```python
from build123d import *

# Parameters (mm, degrees)
BOSS_EXTRUDE1_DEPTH = 18
CUT_EXTRUDE1_DEPTH  = 14
SKETCH5_W           = 38.6
SKETCH5_H           = 4
BOSS_EXTRUDE2_DEPTH = 51.5
SKETCH6_R           = 10
CUT_EXTRUDE2_DEPTH  = 200
SKETCH7_R           = 6
CUT_EXTRUDE3_DEPTH  = 200


with BuildPart() as part:
    # Sketch2 → Boss-Extrude1 (new body)
    with BuildSketch(Plane(origin=(0, 0, 0), x_dir=(1, 0, 0), z_dir=(0, 1, 0))):
        with BuildLine():
            Line((-2.050203312, 17.379489819), (71.229085812, 26.024015225))
            Line((71.229085812, 26.024015225), (70.776256856, -26.027550211))
            Line((70.776256856, -26.027550211), (-2.063605293, -17.37790359))
            ThreePointArc((-2.063605293, -17.37790359), (-17.499998699, 0.006747763), (-2.050203312, 17.379489819))
        make_face()
    extrude(amount=BOSS_EXTRUDE1_DEPTH)

    # Sketch4 → Cut-Extrude1 (cut)
    with BuildSketch(Plane(origin=(0, 18, 0), x_dir=(1, 0, 0), z_dir=(0, 1, 0))):
        with BuildLine():
            Line((35.006766585, 14.999998474), (31.502988077, 14.586668832))
            ThreePointArc((31.502988077, 14.586668832), (20.004544926, -0.369225031), (32.22510993, -14.741098504))
            Line((32.22510993, -14.741098504), (34.245425362, -14.981008548))
            Line((34.245425362, -14.981008548), (70.834558469, -19.325924398))
            Line((70.834558469, -19.325924398), (71.170294461, 19.266095201))
            Line((71.170294461, 19.266095201), (35.006766585, 14.999998474))
        make_face()
    extrude(amount=-CUT_EXTRUDE1_DEPTH, mode=Mode.SUBTRACT)

    # Sketch5 → Boss-Extrude2 (add)
    with BuildSketch(Plane(origin=(70.997313391, 0, 0.617649806), x_dir=(0.008699293, 0, -0.99996216), z_dir=(0.99996216, 0, 0.008699293))):
        with Locations((0.591017469, 16)):
            Rectangle(SKETCH5_W, SKETCH5_H)
    extrude(amount=-BOSS_EXTRUDE2_DEPTH)

    # Sketch6 → Cut-Extrude2 (cut)
    with BuildSketch(Plane(origin=(0, 18, 0), x_dir=(1, 0, 0), z_dir=(0, 1, 0))):
        with Locations((2.500001301, 0)):
            Circle(SKETCH6_R)
    extrude(amount=-CUT_EXTRUDE2_DEPTH, mode=Mode.SUBTRACT)

    # Sketch7 → Cut-Extrude3 (cut)
    with BuildSketch(Plane(origin=(0, 18, 0), x_dir=(1, 0, 0), z_dir=(0, 1, 0))):
        with Locations((35.001789275, 0.053432271)):
            Circle(SKETCH7_R)
        with Locations((55.001789275, 0.053432271)):
            Circle(SKETCH7_R)
    extrude(amount=-CUT_EXTRUDE3_DEPTH, mode=Mode.SUBTRACT)


solid = part.part
```
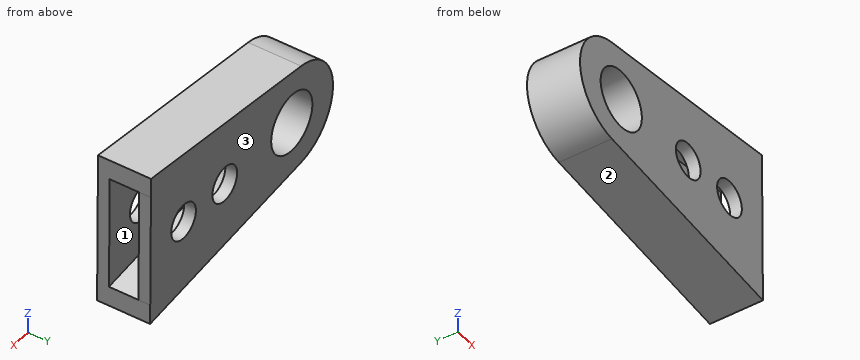
Read the model definition and answer for the solid it produces. Units are mm, in the model's axes. Face numbers are marked on the shaded views. Coordinates: 2 decimals unless noted, no trailing zeros. Loops run counter-clockwise (first coordinate to the right, second up) from the corner with the lowest first, then second, coordinate; pieces in that order, holes last. Notation, with made-up numbers: (60, 80.5) - (116, 80.5) arc R26 ccw to (116, 108.5) - close; hole circle Ø2 at (11, 88). An arc over 180 degrees is marked (long way). Answer in a Markdown table with one row per item.
1. Given pin 1 (8 mm diameter, centred on y = 4, z = 14, fed in from +X); pin 2 (10 mm diameter, centred on x = 36.5, y = 11.5, fed in from +Z); pin 3 (3 mm diameter, centred on x = 35.5, y = 3.5, fed in from +Z), each flat-ended and moving along its own axis, determine where each tip first touches the part or whether it passes through.
Conclusion:
| item | result |
|---|---|
| pin 1 | stops at x = 70.92 |
| pin 2 | stops at z = 22.55 |
| pin 3 | stops at z = 22.02 |
2. Find section C-C, the plane z = -1. Write down the section's boundary in (x, y), then the cut area to 3 significant figures.
Conclusion:
| item | result |
|---|---|
| outline | (-17.47, 0) - (-7.45, 0) - (-7.45, 18) - (-17.47, 18) - close; (12.45, 0) - (29.08, 0) - (29.08, 4) - (20.03, 4) - (20.03, 14) - (29.08, 14) - (29.08, 18) - (12.45, 18) - close; (40.93, 0) - (49.08, 0) - (49.08, 4) - (40.93, 4) - close; (40.93, 14) - (49.08, 14) - (49.08, 18) - (40.93, 18) - close; (60.93, 0) - (71.01, 0) - (71.01, 4) - (60.93, 4) - close; (60.93, 14) - (71.01, 14) - (71.01, 18) - (60.93, 18) - close |
| area | 535 mm² |
3. Find section D-D, the plane y = 15. Write down the section's boundary in (x, z), then the cut area to 3 significant figures.
Conclusion:
| item | result |
|---|---|
| outline | (-2.06, 17.38) arc R17.5 ccw to (-2.05, -17.38) - (71.23, -26.02) - (70.78, 26.03) - close; hole circle Ø20 at (2.5, 0); hole circle Ø12 at (35, -0.05); hole circle Ø12 at (55, -0.05) |
| area | 3,040 mm² |
4. Determine the mould class of the marked faces 1, 2 and 3 for opening direction Y: +Y half, -Y half, draft (parallel to the pull), parting line (faces both ways), or undercut.
Conclusion:
| item | result |
|---|---|
| face 1 | undercut |
| face 2 | draft |
| face 3 | +Y half |
5. Find section A-A, the plane y = 10.25. Write down the section's boundary in (x, z).
Conclusion:
| item | result |
|---|---|
| outline | (-2.06, 17.38) arc R17.5 ccw to (-2.05, -17.38) - (71.23, -26.02) - (71.17, -19.27) - (31.5, -14.59) arc R15 cw to (32.23, 14.74) - (70.83, 19.33) - (70.78, 26.03) - close; hole circle Ø20 at (2.5, 0) |
6. Find section B-B, the plane x = 36.5. Write down the section's boundary in (y, z), then the cut area to 3 significant figures.
Conclusion:
| item | result |
|---|---|
| outline | (0, -21.93) - (18, -21.93) - (18, -5.86) - (14, -5.86) - (14, -15.18) - (4, -15.18) - (4, -5.86) - (0, -5.86) - close; (0, 5.76) - (4, 5.76) - (4, 15.25) - (14, 15.25) - (14, 5.76) - (18, 5.76) - (18, 21.96) - (0, 21.96) - close |
| area | 393 mm² |
7. Straight lines are drawn through the part: line 1 (Y direction, x = 61, z = 18); line 2 (X direction, y = 17, z = 1); line 3 (X direction, y = 17.25, z = -5). For each, find the intervals that lie inside material, in ascending order.
Conclusion:
| item | result |
|---|---|
| line 1 | y = 0 to 4, 14 to 18 |
| line 2 | x = -17.47 to -7.45, 12.45 to 29.09, 40.91 to 49.09, 60.91 to 70.99 |
| line 3 | x = -16.77 to -6.16, 11.16 to 31.61, 38.4 to 51.61, 58.4 to 71.05 |
